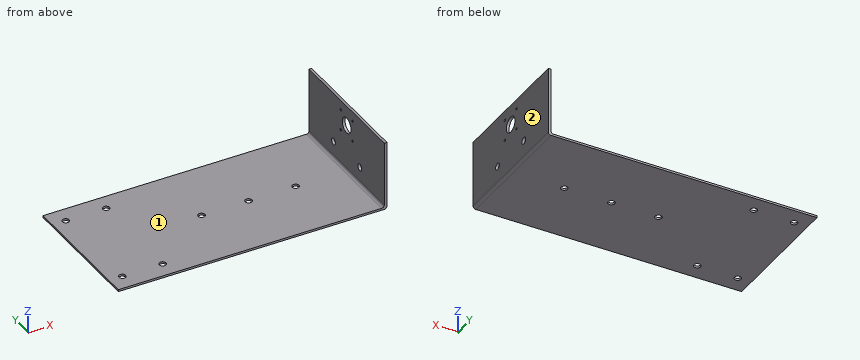
```python
from build123d import *

# Parameters (mm, degrees)
SKETCH1_W           = 400
SKETCH1_H           = 200
BOSS_EXTRUDE1_DEPTH = 3
SKETCH2_R           = 5
CUT_EXTRUDE1_DEPTH  = 10
SKETCH3_W           = 4
SKETCH3_H           = 200
BOSS_EXTRUDE2_DEPTH = 90
FILLET2_R           = 4
SKETCH4_R           = 11.5
CUT_EXTRUDE2_DEPTH  = 90
SKETCH5_R           = 1.75
CUT_EXTRUDE3_DEPTH  = 90
SKETCH6_R           = 5
CUT_EXTRUDE4_DEPTH  = 15
SKETCH7_W           = 4
SKETCH7_H           = 200
BOSS_EXTRUDE3_DEPTH = 10


with BuildPart() as part:
    # Sketch1 → Boss-Extrude1 (new body)
    with BuildSketch(Plane.XY):
        Rectangle(SKETCH1_W, SKETCH1_H)
    extrude(amount=BOSS_EXTRUDE1_DEPTH)

    # Sketch2 → Cut-Extrude1 (cut)
    with BuildSketch(Plane(origin=(0, 0, 0), x_dir=(-1, 0, 0), z_dir=(0, 0, -1))):
        with Locations((-120, 0)):
            Circle(SKETCH2_R)
        with Locations((-50, 0)):
            Circle(SKETCH2_R)
        with Locations((20, 0)):
            Circle(SKETCH2_R)
        with Locations((180, -75)):
            Circle(SKETCH2_R)
        with Locations((120, -75)):
            Circle(SKETCH2_R)
        with Locations((120, 75)):
            Circle(SKETCH2_R)
        with Locations((180, 75)):
            Circle(SKETCH2_R)
    extrude(amount=-CUT_EXTRUDE1_DEPTH, mode=Mode.SUBTRACT)

    # Sketch3 → Boss-Extrude2 (add)
    with BuildSketch(Plane.XY.offset(3)):
        with Locations((198, 0)):
            Rectangle(SKETCH3_W, SKETCH3_H)
    extrude(amount=BOSS_EXTRUDE2_DEPTH)

    # Fillet2
    fillet2_edges = [part.edges().sort_by_distance(p)[0] for p in [
        (196, 0, 3),
        (200, 0, 0),
    ]]
    fillet(fillet2_edges, radius=FILLET2_R)

    # Sketch4 → Cut-Extrude2 (cut)
    with BuildSketch(Plane(origin=(200, 0, 0), x_dir=(0, 0, -1), z_dir=(1, 0, 0))):
        with Locations((-73, 0)):
            Circle(SKETCH4_R)
    extrude(amount=-CUT_EXTRUDE2_DEPTH, mode=Mode.SUBTRACT)

    # Sketch5 → Cut-Extrude3 (cut)
    with BuildSketch(Plane(origin=(200, 0, 0), x_dir=(0, 0, -1), z_dir=(1, 0, 0))):
        with Locations((-57.5, 15.5)):
            Circle(SKETCH5_R)
        with Locations((-57.5, -15.5)):
            Circle(SKETCH5_R)
        with Locations((-88.5, -15.5)):
            Circle(SKETCH5_R)
        with Locations((-88.5, 15.5)):
            Circle(SKETCH5_R)
    extrude(amount=-CUT_EXTRUDE3_DEPTH, mode=Mode.SUBTRACT)

    # Sketch6 → Cut-Extrude4 (cut)
    with BuildSketch(Plane(origin=(200, 0, 0), x_dir=(0, 0, -1), z_dir=(1, 0, 0))):
        with Locations((-28, -35)):
            Circle(SKETCH6_R)
        with Locations((-28, 35)):
            Circle(SKETCH6_R)
    extrude(amount=-CUT_EXTRUDE4_DEPTH, mode=Mode.SUBTRACT)

    # Sketch7 → Boss-Extrude3 (add)
    with BuildSketch(Plane.XY.offset(93)):
        with Locations((198, 0)):
            Rectangle(SKETCH7_W, SKETCH7_H)
    extrude(amount=BOSS_EXTRUDE3_DEPTH)


solid = part.part
```
Part model, mm, in its own coordinate system. Face numbers are marked on the shaded views. A direction names the side the tool comes from. Give positions to 0.01 mm unless a question says otherwise; leave off trailing zeros. Loops run counter-clockwise (first coordinate to the right, second up) from the corner with the lowest first, then second, coordinate; pieces in that order, holes last. Notation, with made-up numbers: M -9.75,4.5 L 18.25,4.5 A20 cw 18.25,23.5 Z; hole C -2,65 d3. An arc over 180 degrees is marked long. Return JSON: item names as keys, results as strings.
1) Saw through at D-D, the plane y = 75. List the corners of the cut face in (x, z), then the cut area to 3 significant figures.
Calculated:
{"outline": "M -200,0 L -185,0 L -185,3 L -200,3 Z; M -175,0 L -125,0 L -125,3 L -175,3 Z; M -115,0 L 196,0 A4 ccw 200,4 L 200,103 L 196,103 L 196,7 A4 cw 192,3 L -115,3 Z", "area": "1,540 mm2"}
2) Saw through at C-C, the plane z = 77.5. List the corners of the cut face in (x, y), then the cut area to 3 significant figures.
Calculated:
{"outline": "M 196,-100 L 200,-100 L 200,-10.58 L 196,-10.58 Z; M 196,10.58 L 200,10.58 L 200,100 L 196,100 Z", "area": "715 mm2"}
3) Flat gauge pins, fed straight in: pin 1 Ø12 at (x, y) = (112, 60.5) entering from +Z; pin 2 Ø5 at (y, z) = (16, 14.5) entering from -X. Where does each tip first touch, or does it go through?
Calculated:
{"pin 1": "stops at z = 3", "pin 2": "stops at x = 196"}
4) 3-axis set-ups, long thin cutter, end or side, ignore diameter. For the marked faces 1 and 2: which of +Z, -Z, +X, -X, +Y, -Y reach the whole face in a straight line?
Calculated:
{"face 1": "+Z, -X, +Y, -Y", "face 2": "+Z, -Z, +X, +Y, -Y"}
5) Drill centre lines: line 1 (Y direction, x = -180, z = 2.2); line 2 (Y direction, x = 198, z = 57); line 3 (Y direction, x = 50, z = 0.7). Where is each one in solid material? Low to high.
Calculated:
{"line 1": "y = -100 to -80, -70 to 70, 80 to 100", "line 2": "y = -100 to -17.18, -13.82 to 13.82, 17.18 to 100", "line 3": "y = -100 to -5, 5 to 100"}
6) Saw through at B-B, the plane y = 0. List the corners of the cut face in (x, z).
Calculated:
{"outline": "M -200,0 L -25,0 L -25,3 L -200,3 Z; M -15,0 L 45,0 L 45,3 L -15,3 Z; M 55,0 L 115,0 L 115,3 L 55,3 Z; M 125,0 L 196,0 A4 ccw 200,4 L 200,61.5 L 196,61.5 L 196,7 A4 cw 192,3 L 125,3 Z; M 196,84.5 L 200,84.5 L 200,103 L 196,103 Z"}
7) Saw through at A-A, the plane x = -120. List the corners of the cut face in (y, z).
Calculated:
{"outline": "M -100,0 L -80,0 L -80,3 L -100,3 Z; M -70,0 L 70,0 L 70,3 L -70,3 Z; M 80,0 L 100,0 L 100,3 L 80,3 Z"}
